Source: CAD feature listing. Evaluate the final solid. Frame: model axes, mm. A direction names the side the tool comes from. Round coordinates to 2 decimals unless told otherwise and drop trailing zeros. Loops run counter-clockwise (first coordinate to the right, second up) from the corner with the lowest first, then second, coordinate; pieces in that order, holes last. Notation, with made-up numbers: (12, 38.25) - (20, 38.25) arc R35 cw to (20, 71.25) - close; hole circle Ø9 at (29, 10). An arc over 180 degrees is marked (long way). One line per question, with ' | ' between items.
from build123d import *

# Parameters (mm, degrees)
SKETCH2_R           = 5
SKETCH2_R_2         = 2.5
BOSS_EXTRUDE1_DEPTH = 10
FILLET1_R           = 10
FILLET2_R           = 3
FILLET3_R           = 3
FILLET4_R           = 3


with BuildPart() as part:
    # Sketch2 → Boss-Extrude1 (new body)
    with BuildSketch(Plane(origin=(0, 0, 0), x_dir=(1, 0, 0), z_dir=(0, 1, 0))):
        with BuildLine():
            Line((66.252272915, -86), (-6, -86))
            Line((-6, -86), (-6, -13.747727085))
            ThreePointArc((-6, -13.747727085), (-5.740251485, 13.858192988), (13.963751735, -5.47847036))
            Line((13.963751735, -5.47847036), (74.52152964, -66.036248265))
            ThreePointArc((74.52152964, -66.036248265), (93.858192988, -85.740251485), (66.252272915, -86))
        make_face()
        Circle(SKETCH2_R, mode=Mode.SUBTRACT)
        with Locations((80, -80)):
            Circle(SKETCH2_R, mode=Mode.SUBTRACT)
        with Locations((50, -80)):
            Circle(SKETCH2_R_2, mode=Mode.SUBTRACT)
        with Locations((24, -80)):
            Circle(SKETCH2_R_2, mode=Mode.SUBTRACT)
        with Locations((0, -56)):
            Circle(SKETCH2_R_2, mode=Mode.SUBTRACT)
        with Locations((0, -30)):
            Circle(SKETCH2_R_2, mode=Mode.SUBTRACT)
        with Locations((28.284271247, -28.284271247)):
            Circle(SKETCH2_R_2, mode=Mode.SUBTRACT)
        with Locations((51.715728753, -51.715728753)):
            Circle(SKETCH2_R_2, mode=Mode.SUBTRACT)
        with Locations((4, -76)):
            Circle(SKETCH2_R_2, mode=Mode.SUBTRACT)
        with BuildLine():
            Line((65.514718626, -74), (18.866068747, -74))
            ThreePointArc((18.866068747, -74), (14.606601718, -65.393398282), (6, -61.133931253))
            Line((6, -61.133931253), (6, -14.485281374))
            Line((6, -14.485281374), (65.514718626, -74))
        make_face(mode=Mode.SUBTRACT)
    extrude(amount=BOSS_EXTRUDE1_DEPTH)

    # Fillet1
    fillet1_edges = [part.edges().sort_by_distance(p)[0] for p in [
        (-6, 5, 86),
    ]]
    fillet(fillet1_edges, radius=FILLET1_R)

    # Fillet2
    fillet2_edges = [part.edges().sort_by_distance(p)[0] for p in [
        (-6, 5, 13.747727085),
        (13.963751735, 5, 5.47847036),
        (74.52152964, 5, 66.036248265),
        (66.252272915, 5, 86),
    ]]
    fillet(fillet2_edges, radius=FILLET2_R)

    # Fillet3
    fillet3_edges = [part.edges().sort_by_distance(p)[0] for p in [
        (65.514718626, 5, 74),
        (6, 5, 14.485281374),
    ]]
    fillet(fillet3_edges, radius=FILLET3_R)

    # Fillet4
    fillet4_edges = [part.edges().sort_by_distance(p)[0] for p in [
        (6, 5, 61.133931253),
        (18.866068747, 5, 74),
    ]]
    fillet(fillet4_edges, radius=FILLET4_R)


solid = part.part
1. Section query B-B, the plane z = 47.5. Return loops of the section in (x, y), plus the area to 3 significant figures.
Worked out:
outline: (-6, 0) - (6, 0) - (6, 10) - (-6, 10) - close; (39.01, 0) - (55.99, 0) - (55.99, 10) - (39.01, 10) - close | area: 290 mm2
2. Section query D-D, the plane y = 6. Give the number of separate pieces and of enclosed holes in the cut face, plus the area to 3 significant figures.
Worked out:
separate pieces: 1 | enclosed holes: 10 | area: 3,820 mm2
3. Section query A-A, the plane x = 80. Return loops of the section in (y, z), plus the area to 3 significant figures.
Worked out:
outline: (0, 65) - (10, 65) - (10, 75) - (0, 75) - close; (0, 85) - (10, 85) - (10, 95) - (0, 95) - close | area: 200 mm2
4. Section query C-C, the plane x = 24. Return loops of the section in (y, z), plus the area to 3 significant figures.
Worked out:
outline: (0, 15.51) - (10, 15.51) - (10, 32.49) - (0, 32.49) - close; (0, 74) - (10, 74) - (10, 77.5) - (0, 77.5) - close; (0, 82.5) - (10, 82.5) - (10, 86) - (0, 86) - close | area: 240 mm2
5. Mould query, pull axis Z, two halves, no side actions, for faces 4 (the flat face through (-6, 5, 46)), 5 (the cylindrical face through (7.806, 5.07, 18.976)), 6 (the flat face through (43.837, 4.93, 35.352)), 7 (the cylindrical face through (5.15, 4.93, 78.22)). Classes: released by +Z, released by -Z, zero draft, split by the parting line, or undercut.
Worked out:
face 4: zero draft | face 5: undercut | face 6: released by -Z | face 7: undercut
6. Access query for faces 1 (the flat face through (35, 5, 86)), 2 (the flat face through (35.412, 4.93, 43.898)), 3 (the cylindrical face through (74.586, 5.07, 65.517)). Directions: +Z, -Z, +X, -X, +Y, -Y. A direction counts if a zero-diameter tool reaches every point of the face in a straight line with its end or side. Return the directions, or none.
Worked out:
face 1: +Z, -X, +Y, -Y | face 2: +Y, -Y | face 3: -Z, +Y, -Y
7. Material intervals for probe 1 along X at (y, z) = (7.75, 0); probe 2 along Z at (x, y) = (0, 3.5); probe 3 along X at (y, z) = (2.5, 79.5), sorted ascending.
Worked out:
probe 1: x = -15 to -5, 5 to 15 | probe 2: z = -15 to -5, 5 to 27.5, 32.5 to 53.5, 58.5 to 85.17 | probe 3: x = -5.37 to 21.55, 26.45 to 47.55, 52.45 to 75.03, 84.97 to 94.99
8. Contact query for flat-ended pins moving along their axis: P1, Ø3, axis at x = 28, y = 3.5, coming from the +Z side; P2, Ø5, axis at x = 9, y = 2.5, coming from the -Z side; P3, Ø5, axis at y = 5.5, z = 47, coming from the +X side. Output: stop coordinate, or through.
Worked out:
P1: stops at z = 86 | P2: stops at z = -13.52 | P3: stops at x = 57.99
